Part print with two shaded views. Sizes in mm from the minimum x, y, z corner. A direction names the side the tool comes from. Give positions to 0.01 mm unless a question says otherwise; leave off trailing zeros. Order: outer loops, then holes, each group sorted by start corner. A loop starts at its lowest first (then second) coordinate and runs counter-clockwise, first axis right, second up. Notation, with made-up numbers: (33.25, 15.5) -> (77.25, 15.5) arc R24 ccw to (77.25, 44.5) -> close; hole circle Ø7 at (-15, 3). An arc over 180 degrees is marked (long way). Write item = value, one per line. Start each with the question number.
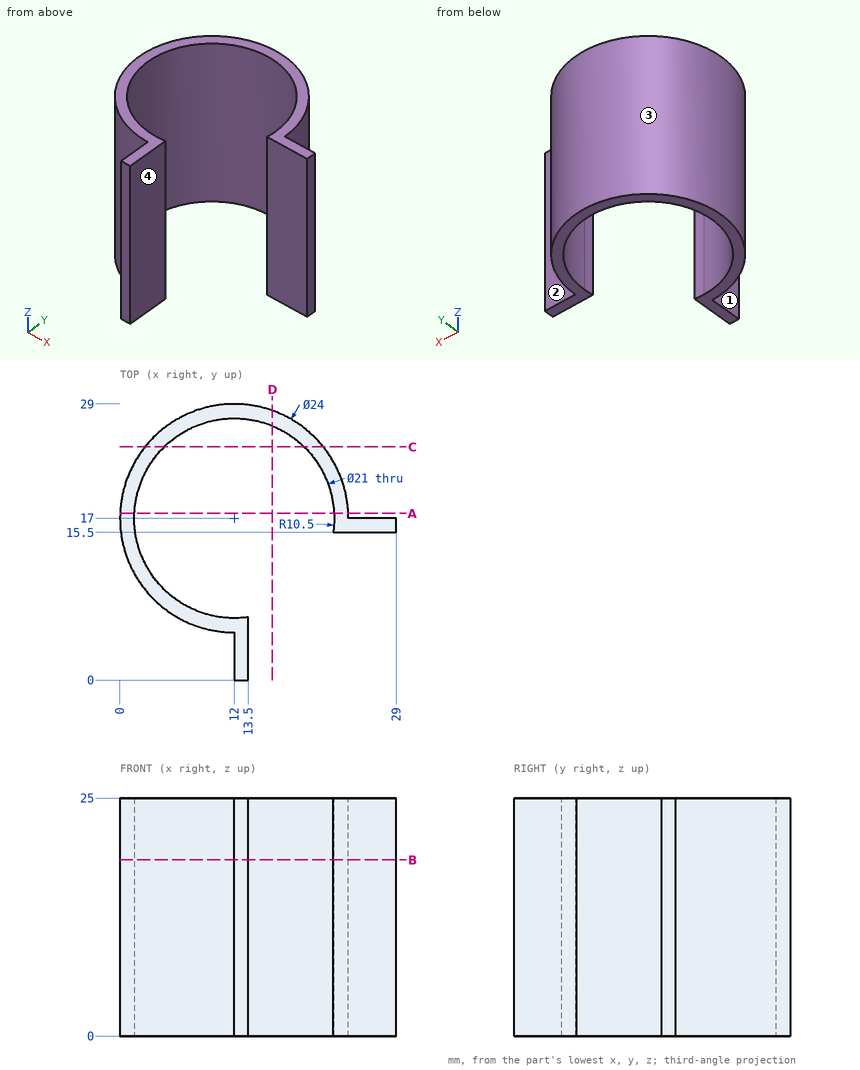
(1) Flat gauge pins, fed straight in: P1, Ø12.5, axis at x = 12, y = 17, coming from the -Z side; P2, Ø2, axis at y = 4, z = 14, coming from the +X side; P3, Ø10, axis at y = 9.5, z = 12.5, coming from the -X side; P4, Ø4, axis at y = 13, z = 13, coming from the +X side. Where does each tip first touch, or does it go through?
(2) Cut at C-C, the plane y = 24.5. Give the cut face in (x, z).
(3) Cut at D-D, the plane x = 16. Give the cut face in (y, z).
(4) Wall check: line 1 (X direction, y = 20.25, z = 17.75); line 2 (X direction, y = 26.5, z = 23.75); line 3 (Y direction, x = 8.5, z = 23). Give the ranges that are in metal, low to high. Write a range as [from, to].
(5) Cut at B-B, the plane z = 18.5. Give the cut face in (x, y).
(6) Cut at A-A, the plane y = 17.5. Give the cut face in (x, z), plus the area to 3 significant figures.
(7) 3-axis set-ups, long thin cutter, end or side, ignore diameter. For the marked faces 1, 2, 3 and 4: which of +Z, -Z, +X, -X, +Y, -Y reach the whole face in a straight line?
Results:
q1.P1 = through
q1.P2 = 13.5
q1.P3 = 0.26
q1.P4 = 3.38
q2.outline = (2.63, 0) -> (4.65, 0) -> (4.65, 25) -> (2.63, 25) -> close; (19.35, 0) -> (21.37, 0) -> (21.37, 25) -> (19.35, 25) -> close
q3.outline = (26.71, 0) -> (28.31, 0) -> (28.31, 25) -> (26.71, 25) -> close
q4.line_1 = [0.45, 2.02], [21.98, 23.55]
q4.line_2 = [4.67, 7.53], [16.47, 19.33]
q4.line_3 = [5.52, 7.1], [26.9, 28.48]
q5.outline = (12, 0) -> (13.5, 0) -> (13.5, 6.61) arc R10.5 cw (long way) to (22.39, 15.5) -> (29, 15.5) -> (29, 17) -> (24, 17) arc R12 ccw (long way) to (12, 5) -> close
q6.outline = (0.01, 0) -> (1.51, 0) -> (1.51, 25) -> (0.01, 25) -> close; (22.49, 0) -> (23.99, 0) -> (23.99, 25) -> (22.49, 25) -> close
q6.area = 75.1 mm2
q7.face_1 = +Z, -Z, -X, -Y
q7.face_2 = +Z, -Z, +X, +Y
q7.face_3 = +Z, -Z
q7.face_4 = +Z, -Z, +X, -Y
